```python
from build123d import *

# Parameters (mm, degrees)
F0_W     = 124
F0_H     = 22
F1_DEPTH = 12
F2_DEPTH = 11
F3_R     = 3
F4_W     = 121.5
F4_H     = 19.5
F5_DEPTH = 9
F6_R     = 0.5


with BuildPart() as f1:
    # F0 (on Top) → F1 (new body)
    with BuildSketch(Plane.XY):
        Rectangle(F0_W, F0_H)
    extrude(amount=F1_DEPTH)

    # F0 (on Top) → F2 (join)
    with BuildSketch(Plane.XY):
        Rectangle(F0_W, F0_H)
    extrude(amount=F2_DEPTH)

    # F3
    f3_edges = [f1.edges().sort_by_distance(p)[0] for p in [
        (0, -11, 0),
        (-62, 0, 0),
        (0, 11, 0),
        (62, 0, 0),
    ]]
    fillet(f3_edges, radius=F3_R)

    # F4 (on face) → F5 (cut)
    with BuildSketch(Plane.XY.offset(12)):
        Rectangle(F4_W, F4_H)
    extrude(amount=-F5_DEPTH, mode=Mode.SUBTRACT)

    # F6
    f6_edges = [f1.edges().sort_by_distance(p)[0] for p in [
        (-62, 11, 7.5),
        (-62, -11, 7.5),
        (62, 11, 7.5),
        (62, -11, 7.5),
    ]]
    fillet(f6_edges, radius=F6_R)


solid = f1.part
```
Model file for the job. Use its own axes, mm. A direction names the side the tool comes from. Coordinates: 2 decimals unless noted, no trailing zeros. Write each loop counter-clockwise with the first axis right and the second up, starting at its lowest first coordinate (ties: lowest second). Pieces come first, ordered by that corner, then holes. Notation, with made-up numbers: (20, 70.5) - (57, 70.5) arc R31 ccw to (57, 95.5) - close; hole circle Ø4 at (4.25, 1.5). An arc over 180 degrees is marked (long way). One line per question, with ' | ' between items. Start each with the question number.
Q1. Cut at A-A, the plane z = 4.5. List the corners of the cut face in (x, y), then the cut area to 3 significant figures.
Q2. Pin check, flat tips, straight feed: pin 1 (5 mm diameter, centred on x = -19.5, y = -7, fed in from +Z); pin 2 (1 mm diameter, centred on y = 4, z = 1.5, fed in from -X). Stop position of each tip, or through.
Q3. Cut at C-C, the plane y = -3.5. List the corners of the cut face in (x, z), then the cut area to 3 significant figures.
Q4. Pull direction Y, two halves, no side cores. Call faces 3 (the face through (0.86, 10.14, 0.9)), 4 (the face through (-62, 0, 7)), 5 (the face through (-60.75, 0, 8)), 6 (the face through (-1, -9.75, 8)): pulls with the +Y half, pulls with the -Y half, needs draft (parallel to the pull), parting line crosses it, or undercut.
Q5. 3-axis set-ups, long thin cutter, end or side, ignore diameter. For faces 1 (the face through (0, 10, 12)), 2 (the face through (60.75, 0, 8)): which of +Z, -Z, +X, -X, +Y, -Y reach the whole face in a straight line?
Q6. Drill centre lines: line 1 (X direction, y = 4, z = 10.5); line 2 (Y direction, x = -36, z = 9); line 3 (Z direction, x = -4.5, y = 2). Where is each one in solid material? Low to high. Write a range as [from, to].
Q7. Cut at B-B, the plane x = -24. List the corners of the cut face in (y, z).
Answer below:
1) outline: (-62, -10.5) arc R0.5 ccw to (-61.5, -11) - (61.5, -11) arc R0.5 ccw to (62, -10.5) - (62, 10.5) arc R0.5 ccw to (61.5, 11) - (-61.5, 11) arc R0.5 ccw to (-62, 10.5) - close; hole (-60.75, -9.75) - (60.75, -9.75) - (60.75, 9.75) - (-60.75, 9.75) - close | area: 359 mm^2
2) pin 1: z = 3 | pin 2: x = -61.83
3) outline: (-62, 3) arc R3 ccw to (-59, 0) - (59, 0) arc R3 ccw to (62, 3) - (62, 12) - (60.75, 12) - (60.75, 3) - (-60.75, 3) - (-60.75, 12) - (-62, 12) - close | area: 391 mm^2
4) face 3: pulls with the +Y half | face 4: needs draft | face 5: undercut | face 6: undercut
5) face 1: +Z, +X, -X, +Y, -Y | face 2: +Z
6) line 1: [-62, -60.75], [60.75, 62] | line 2: [-11, -9.75], [9.75, 11] | line 3: [0, 3]
7) outline: (-11, 3) arc R3 ccw to (-8, 0) - (8, 0) arc R3 ccw to (11, 3) - (11, 12) - (9.75, 12) - (9.75, 3) - (-9.75, 3) - (-9.75, 12) - (-11, 12) - close
